Could you check a few things on this model? Use its own coordinates, in mm. Face numbers are marked on the shaded views. A direction names the side the tool comes from. Give positions to 0.01 mm unless a question says otherwise; leave off trailing zeros. Loops run counter-clockwise (first coordinate to the right, second up) from the corner with the lowest first, then second, coordinate; pieces in that order, holes last. Notation, with made-up numbers: (66, 26) -> (87, 26) arc R15 ccw to (87, 35) -> close; hole circle Ø9 at (1.5, 63.5). An arc over 180 degrees is marked (long way). Put each result on its own line as item: value.
```python
from build123d import *

# Parameters (mm, degrees)
SKETCH1_R           = 12.7
BOSS_EXTRUDE1_DEPTH = 30.1625
SKETCH4_R           = 15.875
BOSS_EXTRUDE2_DEPTH = 50.8
CUT_EXTRUDE1_DEPTH  = 11.176
SKETCH3_R           = 6
CUT_EXTRUDE2_DEPTH  = 8
SKETCH5_R           = 3.175
BOSS_EXTRUDE3_DEPTH = 6.604
CUT_EXTRUDE3_START  = -6.35
SKETCH9_R           = 15.875
SKETCH9_R_2         = 6.35
CUT_EXTRUDE3_DEPTH  = 38.1
FILLET1_R           = 3.175
CHAMFER1_SIZE       = 1.27


with BuildPart() as part:
    # Sketch1 → Boss-Extrude1 (new body)
    with BuildSketch(Plane(origin=(0, 0, 0), x_dir=(1, 0, 0), z_dir=(0, 1, 0))):
        Circle(SKETCH1_R)
    extrude(amount=BOSS_EXTRUDE1_DEPTH)

    # Sketch4 → Boss-Extrude2 (add)
    with BuildSketch(Plane(origin=(0, 30.1625, 0), x_dir=(1, 0, 0), z_dir=(0, 1, 0))):
        Circle(SKETCH4_R)
    extrude(amount=BOSS_EXTRUDE2_DEPTH)

    # Sketch2 → Cut-Extrude1 (cut)
    with BuildSketch(Plane.XZ):
        with BuildLine():
            Line((-7, 2.899494937), (-8.776962921, 1.122532015))
            ThreePointArc((-8.776962921, 1.122532015), (-9.241930906, 0), (-8.776962921, -1.122532015))
            Line((-8.776962921, -1.122532015), (-7, -2.899494937))
            Line((-7, -2.899494937), (-7, 2.899494937))
        make_face()
        Polygon((-2.899494937, 7), (-7, 2.899494937), (-7, -2.899494937), (-2.899494937, -7), (2.899494937, -7), (7, -2.899494937), (7, 2.899494937), (2.899494937, 7), align=None)
        with BuildLine():
            Line((-7, 5.4125), (-7, 2.899494937))
            Line((-7, 2.899494937), (-2.899494937, 7))
            Line((-2.899494937, 7), (-5.4125, 7))
            ThreePointArc((-5.4125, 7), (-6.535032015, 6.535032015), (-7, 5.4125))
        make_face()
        with BuildLine():
            Line((-1.122532015, 8.776962921), (-2.899494937, 7))
            Line((-2.899494937, 7), (2.899494937, 7))
            Line((2.899494937, 7), (1.122532015, 8.776962921))
            ThreePointArc((1.122532015, 8.776962921), (0, 9.241930906), (-1.122532015, 8.776962921))
        make_face()
        with BuildLine():
            Line((5.4125, 7), (2.899494937, 7))
            Line((2.899494937, 7), (7, 2.899494937))
            Line((7, 2.899494937), (7, 5.4125))
            ThreePointArc((7, 5.4125), (6.535032015, 6.535032015), (5.4125, 7))
        make_face()
        with BuildLine():
            Line((8.776962921, 1.122532015), (7, 2.899494937))
            Line((7, 2.899494937), (7, -2.899494937))
            Line((7, -2.899494937), (8.776962921, -1.122532015))
            ThreePointArc((8.776962921, -1.122532015), (9.241930906, 0), (8.776962921, 1.122532015))
        make_face()
        with BuildLine():
            Line((7, -2.899494937), (2.899494937, -7))
            Line((2.899494937, -7), (5.4125, -7))
            ThreePointArc((5.4125, -7), (6.535032015, -6.535032015), (7, -5.4125))
            Line((7, -5.4125), (7, -2.899494937))
        make_face()
        with BuildLine():
            Line((2.899494937, -7), (-2.899494937, -7))
            Line((-2.899494937, -7), (-1.122532015, -8.776962921))
            ThreePointArc((-1.122532015, -8.776962921), (0, -9.241930906), (1.122532015, -8.776962921))
            Line((1.122532015, -8.776962921), (2.899494937, -7))
        make_face()
        with BuildLine():
            Line((-2.899494937, -7), (-7, -2.899494937))
            Line((-7, -2.899494937), (-7, -5.4125))
            ThreePointArc((-7, -5.4125), (-6.535032015, -6.535032015), (-5.4125, -7))
            Line((-5.4125, -7), (-2.899494937, -7))
        make_face()
    extrude(amount=-CUT_EXTRUDE1_DEPTH, mode=Mode.SUBTRACT)

    # Sketch3 → Cut-Extrude2 (cut)
    with BuildSketch(Plane.XZ.offset(-11.176)):
        Circle(SKETCH3_R)
    extrude(amount=-CUT_EXTRUDE2_DEPTH, mode=Mode.SUBTRACT)

    # Sketch5 → Boss-Extrude3 (add)
    with BuildSketch(Plane(origin=(0, 80.9625, 0), x_dir=(1, 0, 0), z_dir=(0, 1, 0))):
        Circle(SKETCH5_R)
    extrude(amount=BOSS_EXTRUDE3_DEPTH)

    # Sketch9 → Cut-Extrude3 (cut)
    with BuildSketch(Plane(origin=(0, 80.9625, 0), x_dir=(1, 0, 0), z_dir=(0, 1, 0)).offset(CUT_EXTRUDE3_START)):
        Circle(SKETCH9_R)
        Circle(SKETCH9_R_2, mode=Mode.SUBTRACT)
    extrude(amount=-CUT_EXTRUDE3_DEPTH, mode=Mode.SUBTRACT)

    # Fillet1
    fillet1_edges = [part.edges().sort_by_distance(p)[0] for p in [
        (-6.35, 36.5125, 0),
        (-6.35, 74.6125, 0),
    ]]
    fillet(fillet1_edges, radius=FILLET1_R)

    # Chamfer1
    chamfer1_edges = [part.edges().sort_by_distance(p)[0] for p in [
        (-15.875, 36.5125, 0),
    ]]
    chamfer(chamfer1_edges, length=CHAMFER1_SIZE)


solid = part.part
```
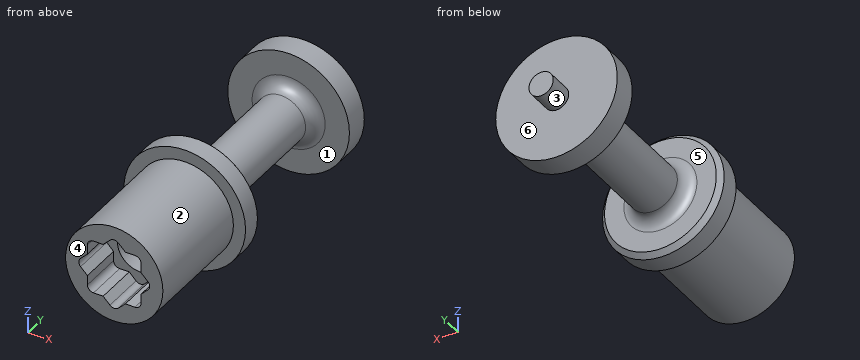
1. I'm going to push flat-ended pins straight in: pin 1 (10 mm diameter, centred on y = 69, z = 9, fed in from -X); pin 2 (1.5 mm diameter, centred on x = -7.5, y = 34.5, fed in from +Z); pin 3 (3 mm diameter, centred on x = -5, y = 3, fed in from -Z). Where does each tip first touch, or does it pass through?
Recorded:
pin 1: stops at x = -4.93
pin 2: stops at z = 14.37
pin 3: stops at z = -12.21
2. Thinking about a two-plate mould opening in Y: for the marked faces 4, 5 and 6, which applies, pulls with the +Y half, pulls with the -Y half, needs draft (parallel to the pull), parting line crosses it, or undercut?
Recorded:
face 4: pulls with the -Y half
face 5: undercut
face 6: pulls with the +Y half
3. If we section it at C-C (y = 61): List the corners of the cut face in (x, z) for me, then the cut area to 3 significant figures.
Recorded:
outline: circle Ø12.7 at (0, 0)
area: 127 mm^2
4. For the marked faces 1, 2 and 3, which set-ups out of +Z, -Z, +X, -X, +Y, -Y let a thin tool reach every point of the face, with its end or its side?
Recorded:
face 1: none
face 2: -Y
face 3: +Y
5. If we section it at D-D (y = 34): List the corners of the cut face in (x, z) for me (3 decimals).
Recorded:
outline: circle Ø31.75 at (0, 0)
6. I need wall thicknesses on line 1 (Z direction, x = 0, y = 13.25); line 2 (Y direction, x = -11, z = -5); line 3 (Y direction, x = 11.5, z = 8). Which ranges of each line are inside material? Lowest first, please.
Recorded:
line 1: z = -12.7 to -6, 6 to 12.7
line 2: y = 0 to 36.51, 74.61 to 80.96
line 3: y = 30.16 to 36.51, 74.61 to 80.96
